Verification items for this drawing (mm, ordinates from the low corner). A direction names the side the tool comes from. Round coordinates to 2 decimals unless told otherwise and drop trailing zeros. Write each loop counter-clockwise with the first axis right and the second up, starting at its lowest first coordinate (ties: lowest second). Pieces come first, ordered by that corner, then holes.
Item 1: Cross-section at B-B (x = 16). Enter the section's corners in (y, z), then the cut area to 3 significant figures.
Item 2: Cross-section at A-A (y = 3). Enter the section's corners in (x, z).
Item 3: Scan lines: probe 1 along Y at (x, z) = (4, 1.3); probe 2 along X at (y, z) = (5, 1); probe 3 along X at (y, z) = (2.5, 1). Record each from-to range of solid material in increasing order.
Item 4: Cross-section at D-D (z = 1.5). Enter the section's corners in (x, y).
Item 5: Depth check by flat-ended pin: P1, Ø1.5, axis at x = 4.5, y = 3.5, coming from the +Z side; P2, Ø1.5, axis at x = 3.5, y = 7, coming from the -Z side; P3, Ø4, axis at x = 28.5, y = 4.5, coming from the +Z side; P4, Ø1, axis at y = 5.5, z = 7.5, coming from the -X side. Enter the tip coordinate at first touch or a pass-through.
Item 6: Draft check along Z on the marked faces 1, 2, 3 and 4. Enter one of: pulls with the +Z half, pulls with the -Z half, needs draft (parallel to the pull), parting line crosses it, or undercut.
Item 7: Cross-section at C-C (z = 6.5). Enter the section's corners in (x, y), then the cut area to 3 significant figures.
Item 8: Access from +Z, -Z, +X, -X, +Y, -Y to the whole of each face (thin tool, end or side, straight path). Record for the marked faces 5 and 6.
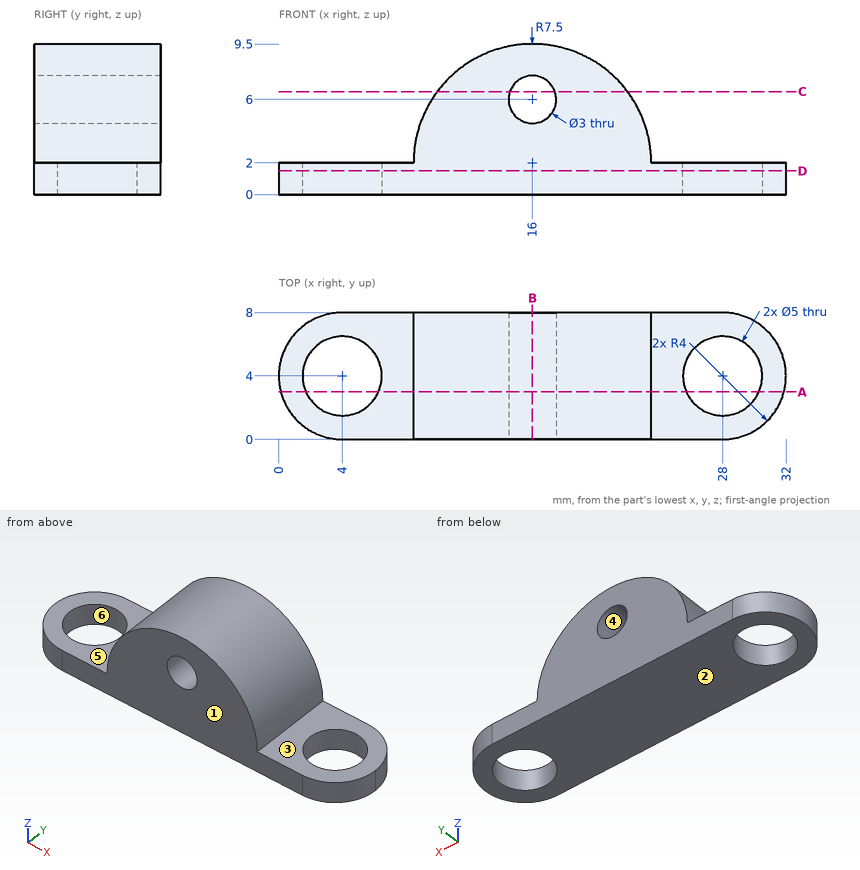
Resolved:
1. outline: (0, 0) - (8, 0) - (8, 4.5) - (0, 4.5) - close; (0, 7.5) - (8, 7.5) - (8, 9.5) - (0, 9.5) - close
1. area: 52.0 mm2
2. outline: (0.13, 0) - (1.71, 0) - (1.71, 2) - (0.13, 2) - close; (6.29, 0) - (25.71, 0) - (25.71, 2) - (23.5, 2) arc R7.5 ccw to (8.5, 2) - (6.29, 2) - close; (30.29, 0) - (31.87, 0) - (31.87, 2) - (30.29, 2) - close; hole circle Ø3 at (16, 6)
3. probe 1: y = 0 to 1.5, 6.5 to 8
3. probe 2: x = 0.13 to 1.71, 6.29 to 25.71, 30.29 to 31.87
3. probe 3: x = 0.29 to 2, 6 to 26, 30 to 31.71
4. outline: (4, 0) - (28, 0) arc R4 ccw to (28, 8) - (4, 8) arc R4 ccw to start; hole circle Ø5 at (4, 4); hole circle Ø5 at (28, 4)
5. P1: passes through
5. P2: stops at z = 0
5. P3: stops at z = 2
5. P4: stops at x = 10.41
6. face 1: needs draft
6. face 2: pulls with the -Z half
6. face 3: pulls with the +Z half
6. face 4: undercut
7. outline: (10, 0) - (14.59, 0) - (14.59, 8) - (10, 8) - close; (17.41, 0) - (22, 0) - (22, 8) - (17.41, 8) - close
7. area: 73.4 mm2
8. face 5: +Z, -X, +Y, -Y
8. face 6: +Z, -Z
